Part print with two shaded views. Sizes in mm from the minimum x, y, z corner. Round coordinates to 2 decimals unless told otherwise and drop trailing zeros. Order: outer loops, then holes, each group sorted by start corner. A loop starts at its lowest first (then second) coordinate and runs counter-clockwise, first axis right, second up. Notation, with made-up numbers: M -3,45.25 L 31,45.25 A17 ccw 31,74.25 Z; hole C -30.5,55.25 d1. An arc over 180 degrees is marked long. Return JSON: item names as keys, results as strings. Group by question number.
Item 1: Slice it at A-A on y = 12.7. Write the cut outline in (x, z), then the cut area to 3 significant figures.
Item 2: Slice it at B-B on z = 3.35. Write the cut outline in (x, y) (3 decimals).
Item 3: Pin check, flat tip, straight feed: pin 1 Ø10 at (x, y) = (48, 21) entering from -Z. Stop position of the tip, or through.
Item 4: Probe line 1 along X through (y, z) = (11.5, 2.25); line 2 along X through (y, z) = (12, 4.4); line 3 along Y through (x, z) = (69, 2.7). List the from-to ranges inside material, lowest first.
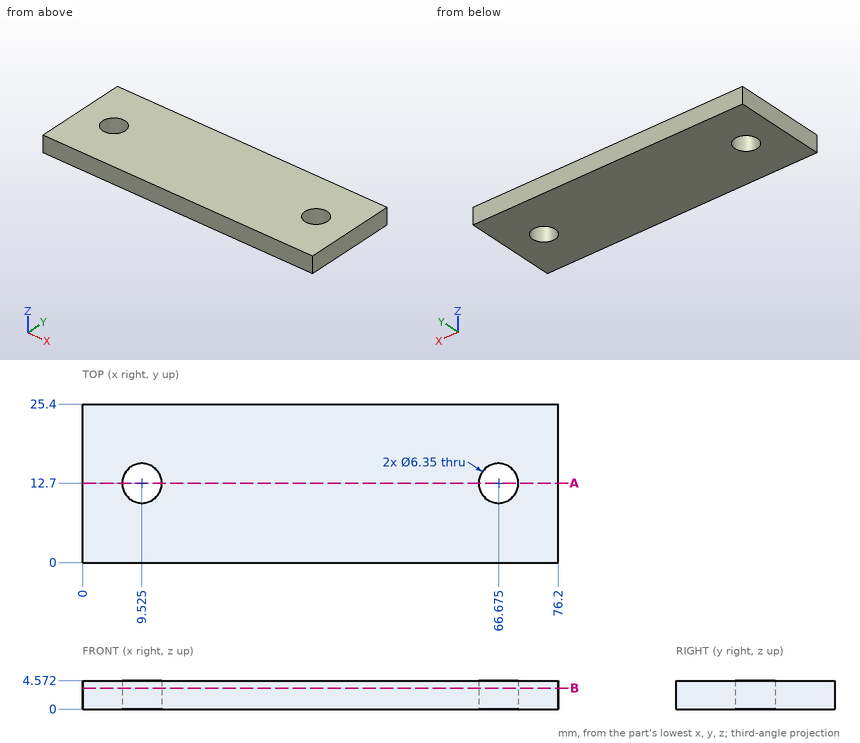
Output values:
{
 "1": {"outline": "M 0,0 L 6.35,0 L 6.35,4.57 L 0,4.57 Z; M 12.7,0 L 63.5,0 L 63.5,4.57 L 12.7,4.57 Z; M 69.85,0 L 76.2,0 L 76.2,4.57 L 69.85,4.57 Z", "area": "290 mm²"},
 "2": {"outline": "M 0,0 L 76.2,0 L 76.2,25.4 L 0,25.4 Z; hole C 9.525,12.7 d6.35; hole C 66.675,12.7 d6.35"},
 "3": {"pin 1": "z = 0"},
 "4": {"line 1": "0 to 6.59, 12.46 to 63.74, 69.61 to 76.2", "line 2": "0 to 6.43, 12.62 to 63.58, 69.77 to 76.2", "line 3": "0 to 10.54, 14.86 to 25.4"}
}
